Input: dimensioned drawing with shaded views. Units: mm. Origin: part minimum x, y, z. A direction names the side the tool comes from. Give positions to 0.01 mm unless a question says otherwise; leave off trailing zeros. Loops run counter-clockwise (first coordinate to the right, second up) from the corner with the lowest first, then second, coordinate; pieces in that order, holes last.
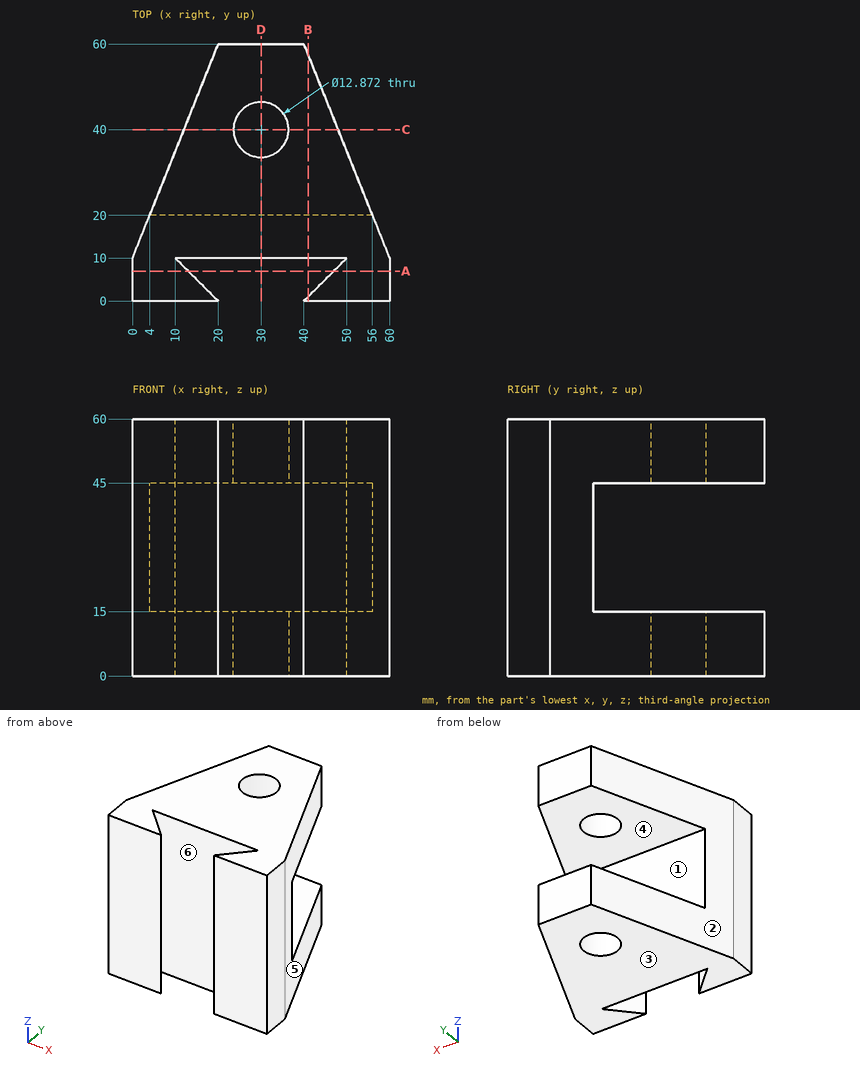
(1) Section D-D, the plane x = 30. Return the cut outline in (y, z), then the cut area to 3 significant figures.
A:
outline: (10, 0) - (33.56, 0) - (33.56, 15) - (20, 15) - (20, 45) - (33.56, 45) - (33.56, 60) - (10, 60) - close; (46.44, 0) - (60, 0) - (60, 15) - (46.44, 15) - close; (46.44, 45) - (60, 45) - (60, 60) - (46.44, 60) - close
area: 1,410 mm2
(2) First-contact query: pin 1 (8 mm diameter, centred on x = 30, z = 6.5, fed in from -Y); pin 2 (12 mm diameter, centred on x = 41.5, z = 36, fed in from +Y); pin 3 (2 mm diameter, centred on y = 39.5, z = 12.5, fed in from -X); pin 4 (12 mm diameter, centred on x = 36.5, z = 39, fed in from -Y). Flat tips, straight axial feed; report the tip coordinate or a pass-through.
A:
pin 1: stops at y = 10
pin 2: stops at y = 20
pin 3: stops at x = 11.4
pin 4: stops at y = 0
(3) Section A-A, the plane y = 7. Return the cut outline in (x, z), then the cut area to 3 significant figures.
A:
outline: (0, 0) - (13, 0) - (13, 60) - (0, 60) - close; (47, 0) - (60, 0) - (60, 60) - (47, 60) - close
area: 1,560 mm2
(4) Mould query, pull axis Z, two halves, no side actions, for the marked faces 1, 2 and 3. Classes: pulls with the +Z half, pulls with the -Z half, needs draft (parallel to the pull), parting line crosses it, or undercut.
A:
face 1: undercut
face 2: needs draft
face 3: pulls with the -Z half
(5) Section B-B, the plane x = 41. Return the cut outline in (y, z), then the cut area to 4 significant figures.
A:
outline: (0, 0) - (1, 0) - (1, 60) - (0, 60) - close; (10, 0) - (57.5, 0) - (57.5, 15) - (20, 15) - (20, 45) - (57.5, 45) - (57.5, 60) - (10, 60) - close
area: 1,785 mm2
(6) Section C-C, the plane y = 40. Return the cut outline in (x, z), then the cut area to 3 significant figures.
A:
outline: (12, 0) - (23.56, 0) - (23.56, 15) - (12, 15) - close; (12, 45) - (23.56, 45) - (23.56, 60) - (12, 60) - close; (36.44, 0) - (48, 0) - (48, 15) - (36.44, 15) - close; (36.44, 45) - (48, 45) - (48, 60) - (36.44, 60) - close
area: 694 mm2
(7) Ray query, line 1 along Y through (x, z) = (30, 50.5); line 2 along Z through (x, y) = (40, 33); line 3 along Y through (x, z) = (47.5, 19). Return the intervals inside material, ascending.
A:
line 1: y = 10 to 33.56, 46.44 to 60
line 2: z = 0 to 15, 45 to 60
line 3: y = 0 to 7.5, 10 to 20
(8) Reachability of the marked faces 4, 5 and 6 from +Z, -Z, +X, -X, +Y, -Y: full face, straight path, thin tool, end or side. Return the list, or none.
A:
face 4: +X, -X, +Y
face 5: +Z, -Z, +X, +Y
face 6: +Z, -Z
